CAD build for the part. Positions are in the model's coordinates, mm. A direction names the side the tool comes from. Give positions to 0.01 mm unless a question says otherwise; leave off trailing zeros. Loops run counter-clockwise (first coordinate to the right, second up) from the corner with the lowest first, then second, coordinate; pieces in that order, holes last. Notation, with made-up numbers: (-29, 59) - (18, 59) arc R16 cw to (18, 89) - close; hole circle Ø7 at (75, 16.25). An arc over 180 degrees is marked (long way). Return JSON: item names as keys, results as strings.
from build123d import *
from build123d import SkipClean  # not in build123d's __all__

# Parameters (mm, degrees)
F0_W      = 50.8
F0_H      = 31.75
F1_DEPTH  = 6.35
F2_W      = 50.8
F2_H      = 12.7
F3_DEPTH  = 44.45
F4_R      = 12.7
F5_DEPTH  = 12.7
F6_R      = 6.35
F7_DEPTH  = 12.7
F8_R      = 3.175
F9_DEPTH  = 25.4
F11_DEPTH = 25.4
F13_DEPTH = 25.4


with BuildPart() as f1:
    # F0 (on Top) → F1 (new body)
    with BuildSketch(Plane.XY):
        with Locations((25.4, 15.875)):
            Rectangle(F0_W, F0_H)
    extrude(amount=F1_DEPTH)

    # F2 (on face) → F3 (join)
    with BuildSketch(Plane.XY.offset(6.35)):
        with Locations((25.4, 25.4)):
            Rectangle(F2_W, F2_H)
    extrude(amount=F3_DEPTH)

    # F4 (on face) → F5 (join)
    with BuildSketch(Plane.XZ.offset(-19.05)):
        with Locations((25.4, 37.9059378386)):
            Circle(F4_R)
    extrude(amount=F5_DEPTH)

    # F6 (on face) → F7 (cut)
    with BuildSketch(Plane.XZ.offset(-6.35)):
        with Locations((25.4, 37.9059378386)):
            Circle(F6_R)
    extrude(amount=-F7_DEPTH, mode=Mode.SUBTRACT)

    # F8 (on face) → F9 (cut)
    with BuildSketch(Plane.XY.offset(6.35)):
        with Locations((5.8808145113, 9.525)):
            Circle(F8_R)
        with Locations((43.9513325691, 9.525)):
            Circle(F8_R)
    extrude(amount=-F9_DEPTH, mode=Mode.SUBTRACT)

    # F10 (on face) → F11 (cut)
    with BuildSketch(Plane.XY.offset(6.35)):
        with BuildLine():
            ThreePointArc((50.8, 6.35), (48.9094635793, 1.8905364207), (44.45, 0))
            Line((44.45, 0), (50.8, 0))
            Line((50.8, 0), (50.8, 6.35))
        make_face()
        with BuildLine():
            ThreePointArc((6.35, 0), (1.9050641376, 1.9050641376), (0, 6.35))
            Line((0, 6.35), (0, 0))
            Line((0, 0), (6.35, 0))
        make_face()
    extrude(amount=-F11_DEPTH, mode=Mode.SUBTRACT)

    # F12 (on face) → F13 (cut)
    with BuildSketch(Plane.XZ.offset(-19.05)):
        with BuildLine():
            ThreePointArc((38.1, 37.9059378386), (38.084216594, 37.2729691208), (38.0369056067, 36.6415736948))
            Line((38.0369056067, 36.6415736948), (38.0369056067, 12.7))
            ThreePointArc((38.0369056067, 12.7), (43.6722535382, 8.0251871407), (50.8, 6.35))
            Line((50.8, 6.35), (50.8, 50.8))
            Line((50.8, 50.8), (0, 50.8))
            Line((0, 50.8), (0, 6.35))
            ThreePointArc((0, 6.35), (7.1277464618, 8.0251871407), (12.7630943933, 12.7))
            Line((12.7630943933, 12.7), (12.7630943933, 36.6415736948))
            ThreePointArc((12.7630943933, 36.6415736948), (24.7670312823, 50.5901544325), (38.1, 37.9059378386))
        make_face()
    with SkipClean():  # cleaning this boolean's faces spoils the solid; the shape is the same uncleaned
        extrude(amount=-F13_DEPTH, mode=Mode.SUBTRACT)


solid = f1.part
1. Pull direction X, two halves, no side cores. Call faces 6 (the face through (43.58, 25.31, 8.07)), 7 (the face through (25, 19.05, 38)), 8 (the face through (1.95, 1.86, 3.22)): +X half, -X half, draft (parallel to the pull), parting line (faces both ways), or undercut.
Values follow:
{"face 6": "+X half", "face 7": "undercut", "face 8": "-X half"}
2. Cut at A-A, the plane y = 11. Write the cut outline in (x, z).
Values follow:
{"outline": "(0, 0) - (3.07, 0) - (3.07, 6.35) - (0, 6.35) - close; (8.69, 0) - (41.14, 0) - (41.14, 6.35) - (8.69, 6.35) - close; circle Ø25.4 at (25.4, 37.91); (46.76, 0) - (50.8, 0) - (50.8, 6.35) - (46.76, 6.35) - close; hole circle Ø12.7 at (25.4, 37.91)"}
3. Which spindle directions (+Z, -Z, +X, -X, +Y, -Y) get a long thin tool onto all of the face, cutting with end or side? Do faces 1 (the face through (12.763, 25, 25)), 2 (the face through (28, 6.35, 44)), 3 (the face through (20.72, 12.61, 42.2)), 4 (the face through (38.037, 25, 25)), 5 (the face through (25, 10, 6.35)). Say none if no direction does.
Values follow:
{"face 1": "-X, +Y, -Y", "face 2": "+Z, +X, -X, -Y", "face 3": "-Y", "face 4": "+X, +Y, -Y", "face 5": "+X, -X, -Y"}
4. Drill centre lines: probe 1 along Z at (x, y) = (29, 11.5); probe 2 along Z at (x, y) = (42, 19); probe 3 along X at (y, z) = (21, 28). Where is each one in solid material? Low to high.
Values follow:
{"probe 1": "z = 0 to 6.35, 25.73 to 32.68, 43.14 to 50.09", "probe 2": "z = 0 to 6.35", "probe 3": "x = 12.76 to 38.04"}
5. Cut at C-C, the plane x = 5. Write the cut outline in (y, z).
Values follow:
{"outline": "(0.18, 0) - (6.47, 0) - (6.47, 6.35) - (0.18, 6.35) - close; (12.58, 0) - (31.75, 0) - (31.75, 7.15) - (19.05, 7.15) - (19.05, 6.35) - (12.58, 6.35) - close"}
6. Cut at D-D, the plane y = 21.5. Write the cut outline in (x, z), plus the area to 3 significant figures.
Values follow:
{"outline": "(0, 0) - (50.8, 0) - (50.8, 6.35) arc R16 cw to (38.04, 12.7) - (38.04, 36.64) arc R12.7 ccw (long way) to (12.76, 36.64) - (12.76, 12.7) arc R16 cw to (0, 6.35) - close", "area": "1,420 mm²"}
7. Cut at B-B, the plane y = 15. Write the cut outline in (x, z).
Values follow:
{"outline": "(0, 0) - (50.8, 0) - (50.8, 6.35) - (0, 6.35) - close; circle Ø25.4 at (25.4, 37.91); hole circle Ø12.7 at (25.4, 37.91)"}
8. Drop flat-ended pins along their axis: P1, Ø10, axis at y = 25.5, z = 27.5, coming from the -X side; P2, Ø5.5, axis at x = 33, y = 8.5, coming from the +Z side; P3, Ø4, axis at y = 9.5, z = 28.5, coming from the +X side; P4, Ø10, axis at x = 17, y = 7, coming from the -Z side. Give the stop position or say it passes through.
Values follow:
{"P1": "stops at x = 12.76", "P2": "stops at z = 49.64", "P3": "stops at x = 35.72", "P4": "stops at z = 0"}
